Part model, mm, in its own coordinate system. Face numbers are marked on the shaded views. A direction names the side the tool comes from. Coordinates: 2 decimals unless noted, no trailing zeros. Order: outer loops, then holes, each group sorted by start corner. A loop starts at its lowest first (then second) coordinate and runs counter-clockwise, first axis right, second up. Notation, with made-up numbers: M -26,37 L -7,37 A24 cw -7,59 Z; hole C 52.5,-22 d4. An arc over 180 degrees is marked long. Write item = value, one per line. Start each with the question number.
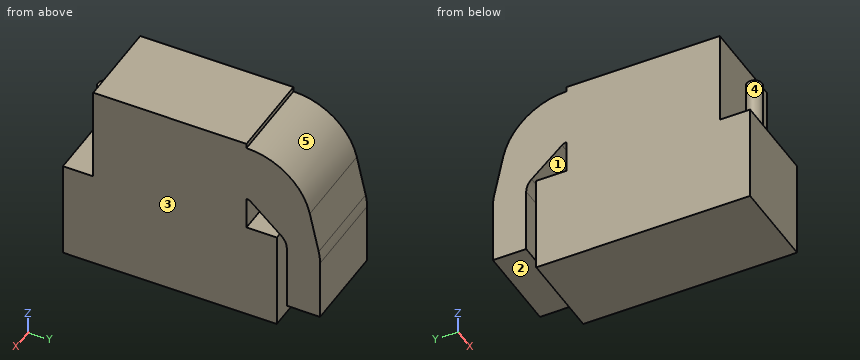
from build123d import *

# Parameters (mm, degrees)
PAD015_DEPTH = 14
SKETCH019_R  = 1.2
SKETCH019_W  = 24
SKETCH019_H  = 13
PAD014_DEPTH = 16
BOX068_W     = 14
BOX068_H     = 24
BOX068_DEPTH = 29.5
BOX067_W     = 14
BOX067_H     = 33.5
BOX067_DEPTH = 15.5


with BuildPart() as pad015:
    # Sketch020 → Pad015 (new body)
    with BuildSketch(Plane.YZ.offset(-232)):
        with BuildLine():
            Line((58.746344, 151.629037), (56.780618, 151.629037))
            Line((56.780618, 151.629037), (56.780618, 160.732927))
            Line((56.780618, 160.732927), (58.746348, 160.732927))
            ThreePointArc((68.674081, 152.764142), (65.111515, 158.494314), (58.746348, 160.732927))
            Line((70.065189, 146.485826), (68.674081, 152.764142))
            ThreePointArc((70.282905, 144.496813), (70.228314, 145.49726), (70.065189, 146.485826))
            Line((70.282905, 134.870576), (70.282905, 144.496813))
            Line((65.069016, 134.870576), (70.282905, 134.870576))
            Line((65.069016, 145.176214), (65.069016, 134.870576))
            ThreePointArc((65.069016, 145.176214), (64.846538, 146.220855), (64.217716, 147.084195))
            Line((59.457466, 151.35671), (64.217716, 147.084195))
            ThreePointArc((59.457466, 151.35671), (59.127086, 151.558628), (58.746344, 151.629037))
        make_face()
    extrude(amount=-PAD015_DEPTH)


with BuildPart() as pad014:
    # Sketch019 → Pad014 (new body)
    with BuildSketch(Plane(origin=(-119, 23.5, 141), x_dir=(0, 1, 0), z_dir=(0, 0, 1))):
        with Locations((37, 120)):
            Circle(SKETCH019_R)
        with Locations((9.5, 120)):
            Circle(SKETCH019_R)
        with Locations((23.25, 120)):
            Rectangle(SKETCH019_W, SKETCH019_H)
    extrude(amount=PAD014_DEPTH)


with BuildPart() as cubo014:
    # Box068 → Box068 (new body)
    with BuildSketch(Plane(origin=(-246, 34.75, 132), x_dir=(1, 0, 0), z_dir=(0, 0, 1))):
        with Locations((7, 12)):
            Rectangle(BOX068_W, BOX068_H)
    extrude(amount=BOX068_DEPTH)


with BuildPart() as head_positive_cut:
    # Box067 → Box067 (new body)
    with BuildSketch(Plane(origin=(-246, 30, 131), x_dir=(1, 0, 0), z_dir=(0, 0, 1))):
        with Locations((7, 16.75)):
            Rectangle(BOX067_W, BOX067_H)
    extrude(amount=BOX067_DEPTH)

    # Fusion065: union Pad015, Pad014, Cubo014
    add(pad015.part)
    add(pad014.part)
    add(cubo014.part)


solid = head_positive_cut.part
Item 1: Cut at B-B, the plane y = 33. Write the cut outline in (x, z), and give its area (3 significant figures).
Item 2: Cut at D-D, the plane z = 148. Write the cut outline in (x, y), and give its area (4 significant figures).
Item 3: Flat gauge pins, fed straight in: pin 1 (4 mm diameter, centred on x = -235.5, y = 67, fed in from -Z); pin 2 (4 mm diameter, centred on x = -238.5, y = 32.5, fed in from +Z); pin 3 (1.5 mm diameter, centred on x = -236, z = 150, fed in from +Y). Where does each tip first touch, or does it go through?
Item 4: 3-axis set-ups, long thin cutter, end or side, ignore diameter. For the marked faces 4 and 5: which of +Z, -Z, +X, -X, +Y, -Y reach the whole face in a straight line?
Item 5: Pull direction Z, two halves, no side cores. Call the marked faces 1, 2 and 3: pulls with the +Z half, pulls with the -Z half, needs draft (parallel to the pull), parting line crosses it, or undercut.
Item 6: Cut at C-C, the plane x = -235.25. Write the cut outline in (y, z), and give its area (3 significant figures).
Item 7: Cut at A-A, the plane z = 140. Write the cut outline in (x, y), and give its area (3 significant figures).
Item 8: Wall check: line 1 along Y through (x, z) = (-241, 138); line 2 along X through (y, z) = (33, 155); line 3 along Y through (x, z) = (-233.5, 147.5). Give the ranges that are in metal, low to high. Write a range as [from, to].
Filled sheet:
q1.outline = M -246,131 L -232,131 L -232,146.5 L -237.8,146.5 L -237.8,157 L -240.2,157 L -240.2,146.5 L -246,146.5 Z
q1.area = 242 mm2
q2.outline = M -246,34.75 L -232,34.75 L -232,58.75 L -246,58.75 Z; M -246,63.2 L -232,63.2 L -232,69.73 L -246,69.73 Z; C -239,33 d2.4; C -239,60.5 d2.4
q2.area = 436.5 mm2
q3.pin_1 = 134.87
q3.pin_2 = 157
q3.pin_3 = 69.45
q4.face_4 = +Z
q4.face_5 = +Z, +X, -X, +Y
q5.face_1 = undercut
q5.face_2 = pulls with the -Z half
q5.face_3 = needs draft
q6.outline = M 30,131 L 63.5,131 L 63.5,146.5 L 58.75,146.5 L 58.75,151.63 A1.06 cw 59.46,151.36 L 64.22,147.08 A2.56 cw 65.07,145.18 L 65.07,134.87 L 70.28,134.87 L 70.28,144.5 A9.19 ccw 70.07,146.49 L 68.67,152.76 A10.17 ccw 58.75,160.73 L 58.75,161.5 L 34.75,161.5 L 34.75,146.5 L 30,146.5 Z
q6.area = 1,050 mm2
q7.outline = M -246,30 L -232,30 L -232,63.5 L -246,63.5 Z; M -246,65.07 L -232,65.07 L -232,70.28 L -246,70.28 Z
q7.area = 542 mm2
q8.line_1 = [30, 63.5], [65.07, 70.28]
q8.line_2 = [-240.2, -237.8]
q8.line_3 = [34.75, 58.75], [63.75, 69.84]
